Design review of the part built by this model. Coordinates are the model's own, in mm. A direction names the side the tool comes from. Give positions to 0.01 mm unless a question says otherwise; leave off trailing zeros. Loops run counter-clockwise (first coordinate to the right, second up) from the corner with the lowest first, then second, coordinate; pieces in that order, holes last.
from build123d import *

# Parameters (mm, degrees)
F1_DEPTH = 25.4
F2_R     = 3.429
F3_DEPTH = 82.551
F4_R     = 3.429
F5_DEPTH = 171.451
F6_W     = 25.4
F6_H     = 25.4
F6_R     = 3.429
F7_DEPTH = 171.451
F8_R     = 3.429
F9_DEPTH = 171.451


with BuildPart() as f1:
    # F0 (on Front) → F1 (new body)
    with BuildSketch(Plane.XZ):
        with BuildLine():
            Line((3.03784, 171.45), (0, 171.45))
            Line((0, 171.45), (0, 5.57784))
            ThreePointArc((0, 5.57784), (1.633712, 1.633712), (5.57784, 0))
            Line((5.57784, 0), (82.55, 0))
            Line((82.55, 0), (82.55, 3.03784))
            Line((82.55, 3.03784), (5.57784, 3.03784))
            ThreePointArc((5.57784, 3.03784), (3.781789, 3.781789), (3.03784, 5.57784))
            Line((3.03784, 5.57784), (3.03784, 171.45))
        make_face()
    extrude(amount=F1_DEPTH)

    # F2 (on face) → F3 (cut, through all)
    with BuildSketch(Plane(origin=(0, 0, 0), x_dir=(0, -1, 0), z_dir=(-1, 0, 0))):
        with BuildLine():
            ThreePointArc((16.129, 154.94), (12.7, 158.369), (9.271, 154.94))
            Line((9.271, 154.94), (9.271, 146.05))
            ThreePointArc((9.271, 146.05), (12.7, 142.621), (16.129, 146.05))
            Line((16.129, 146.05), (16.129, 154.94))
        make_face()
        with Locations((12.7, 82.55)):
            Circle(F2_R)
        with Locations((12.7, 59.69)):
            Circle(F2_R)
    extrude(amount=-F3_DEPTH, mode=Mode.SUBTRACT)

    # F4 (on face) → F5 (cut, through all)
    with BuildSketch(Plane(origin=(0, 0, 0), x_dir=(1, 0, 0), z_dir=(0, 0, -1))):
        with Locations((25.4, 12.7)):
            Circle(F4_R)
        with Locations((69.85, 12.7)):
            Circle(F4_R)
    extrude(amount=-F5_DEPTH, mode=Mode.SUBTRACT)

    # F6 (on face) → F7 (cut, through all)
    with BuildSketch(Plane(origin=(0, 0, 0), x_dir=(1, 0, 0), z_dir=(0, 0, -1))):
        with Locations((69.85, 12.7)):
            Rectangle(F6_W, F6_H)
        with Locations((69.85, 12.7)):
            Circle(F6_R, mode=Mode.SUBTRACT)
    extrude(amount=-F7_DEPTH, mode=Mode.SUBTRACT)

    # F8 (on face) → F9 (cut, through all)
    with BuildSketch(Plane(origin=(0, 0, 0), x_dir=(1, 0, 0), z_dir=(0, 0, -1))):
        with Locations((49.2125, 12.7)):
            Circle(F8_R)
    extrude(amount=-F9_DEPTH, mode=Mode.SUBTRACT)


solid = f1.part
Q1. Draft analysis for pull direction Y (two halves, no side actions). For faces 1 (the face through (32, -13, 3.038)), 2 (the face through (1, 0, 86)), 3 (the face through (1.5, -12.62, 142.62)), state which applies: pulls with the +Y half, pulls with the -Y half, needs draft (parallel to the pull), parting line crosses it, or undercut.
Results:
face 1: needs draft
face 2: pulls with the +Y half
face 3: undercut
Q2. Tool access review of faces 4 (the face through (3.038, -13, 87)), 5 (the face through (48.469, -9.353, 1.498)), 6 (the face through (1, -9.271, 151)): name each direction out of +Z, -Z, +X, -X, +Y, -Y from which nothing blocks a thin tool from reaching the whole face with its end or side.
Results:
face 4: +Z, +X, +Y, -Y
face 5: +Z, -Z
face 6: +X, -X
Q3. Insertion check: pin 1 (10 mm diameter, centred on y = -4.5, z = 88.5, fed in from +X); pin 2 (7.5 mm diameter, centred on x = 40.5, y = -12.5, fed in from +Z). Each pin has a flat end and moves straight along its axis. Give the tip position at first contact, or say it passes through.
Results:
pin 1: stops at x = 3.04
pin 2: stops at z = 3.04
Q4. Take a section at D-D (y = -5). Give the boundary of the cut face in (x, z).
Results:
outline: (0, 5.58) arc R5.58 ccw to (5.58, 0) - (57.15, 0) - (57.15, 3.04) - (5.58, 3.04) arc R2.54 cw to (3.04, 5.58) - (3.04, 171.45) - (0, 171.45) - close
Q5. Take a section at C-C (z = 59.69). Give the boundary of the cut face in (x, y).
Results:
outline: (0, -25.4) - (3.04, -25.4) - (3.04, -16.13) - (0, -16.13) - close; (0, -9.27) - (3.04, -9.27) - (3.04, 0) - (0, 0) - close
Q6. Wall thickness on line 1 (X direction, y = -12.7, z = 2.1); line 2 (Z direction, x = 1.4, y = -12.7); line 3 (Y direction, x = 25.4, z = 2.1): over which ranges is each line inside the solid? List them lowest first.
Results:
line 1: x = 1.22 to 21.97, 28.83 to 45.78, 52.64 to 57.15
line 2: z = 1.88 to 56.26, 63.12 to 79.12, 85.98 to 142.62, 158.37 to 171.45
line 3: y = -25.4 to -16.13, -9.27 to 0
Q7. Take a section at B-B (y = -12.7). Give the boundary of the cut face in (x, z).
Results:
outline: (0, 5.58) arc R5.58 ccw to (5.58, 0) - (21.97, 0) - (21.97, 3.04) - (5.58, 3.04) arc R2.54 cw to (3.04, 5.58) - (3.04, 56.26) - (0, 56.26) - close; (0, 63.12) - (3.04, 63.12) - (3.04, 79.12) - (0, 79.12) - close; (0, 85.98) - (3.04, 85.98) - (3.04, 142.62) - (0, 142.62) - close; (0, 158.37) - (3.04, 158.37) - (3.04, 171.45) - (0, 171.45) - close; (28.83, 0) - (45.78, 0) - (45.78, 3.04) - (28.83, 3.04) - close; (52.64, 0) - (57.15, 0) - (57.15, 3.04) - (52.64, 3.04) - close
Q8. Take a section at A-A (x = 25.4). Give the boundary of the cut face in (y, z).
Results:
outline: (-25.4, 0) - (-16.13, 0) - (-16.13, 3.04) - (-25.4, 3.04) - close; (-9.27, 0) - (0, 0) - (0, 3.04) - (-9.27, 3.04) - close
